```python
from build123d import *

# Parameters (mm, degrees)
F0_W     = 38.862
F0_H     = 38.862
F0_W_2   = 34.862
F0_H_2   = 34.862
F1_DEPTH = 97
F2_DEPTH = 2


with BuildPart() as f1:
    # F0 (on Top) → F1 (new body)
    with BuildSketch(Plane.XY):
        Rectangle(F0_W, F0_H)
        Rectangle(F0_W_2, F0_H_2, mode=Mode.SUBTRACT)
    extrude(amount=F1_DEPTH)

    # F0 (on Top) → F2 (join)
    with BuildSketch(Plane.XY):
        Rectangle(F0_W, F0_H)
        Rectangle(F0_W_2, F0_H_2, mode=Mode.SUBTRACT)
        Rectangle(F0_W_2, F0_H_2)
    extrude(amount=-F2_DEPTH)


solid = f1.part
```
Design review of the part built by this model. Coordinates are the model's own, in mm. A direction names the side the tool comes from. Round coordinates to 2 decimals unless told otherwise and drop trailing zeros. Order: outer loops, then holes, each group sorted by start corner. A loop starts at its lowest first (then second) coordinate and runs counter-clockwise, first axis right, second up. Notation, with made-up numbers: M 82.25,51.25 L 94.25,51.25 A24 ccw 94.25,73.25 Z; hole C 45.5,86 d5. An arc over 180 degrees is marked long. Put each result on its own line as item: value.
Q1. Insertion check: pin 1 Ø3 at (x, y) = (1, -1) entering from +Z. The pin has a flat end and moves straight along its axis. Give the tip position at first contact, or say it passes through.
Reported:
pin 1: z = 0
Q2. To check wall thickness, follow line 1 (X direction, y = 13, z = 27.5); line 2 (Z direction, x = 1.5, y = 6). State the ranges of each line that lie inside material, in increasing order.
Reported:
line 1: -19.43 to -17.43, 17.43 to 19.43
line 2: -2 to 0
Q3. Draft analysis for pull direction X (two halves, no side actions). For faces 1 (the face through (-17.431, 0, 48)), 2 (the face through (-19.431, 0, 48)), 3 (the face through (-2, -19, 97)), state which applies: released by +X, released by -X, zero draft, split by the parting line, or undercut.
Reported:
face 1: undercut
face 2: released by -X
face 3: zero draft
Q4. Machinability: for faces 4 (the face through (0, 0, -2)), 5 (the face through (0, 0, 0)), which of the approach directions +Z, -Z, +X, -X, +Y, -Y give a long, thin tool a straight path to every point of the face, cutting with its end or side? Answer none if there is none.
Reported:
face 4: -Z, +X, -X, +Y, -Y
face 5: +Z
Q5. Consider section B-B (x = 11.5). State the section outline as (y, z) points, and give its area (3 significant figures).
Reported:
outline: M -19.43,-2 L 19.43,-2 L 19.43,97 L 17.43,97 L 17.43,0 L -17.43,0 L -17.43,97 L -19.43,97 Z
area: 466 mm²
Q6. Consider section A-A (z = 37.5). State the section outline as (x, y) points.
Reported:
outline: M -19.43,-19.43 L 19.43,-19.43 L 19.43,19.43 L -19.43,19.43 Z; hole M -17.43,-17.43 L 17.43,-17.43 L 17.43,17.43 L -17.43,17.43 Z
